Work out the finished part from the listing and answer in its coordinate system (mm). Give positions to 0.01 mm unless a question says otherwise; leave off trailing zeros. Loops run counter-clockwise (first coordinate to the right, second up) from the corner with the lowest first, then second, coordinate; pieces in that order, holes last. Notation, with made-up numbers: M 64.25,-34 L 99.25,-34 A12 cw 99.25,-29 Z; hole C 23,12 d1. An arc over 180 degrees is marked long. Use a Markdown table: item, result.
```python
from build123d import *

# Parameters (mm, degrees)
SKETCH1_R               = 19.05
BOSS_EXTRUDE1_DEPTH     = 1524
SHELL1_T                = -2.54
CUT_EXTRUDE1_DEPTH      = 127
CUT_EXTRUDE1_DEPTH_BACK = 127
SKETCH2_OUTSIDE_W       = 1830.99
SKETCH2_OUTSIDE_H       = 345.09


with BuildPart() as part:
    # Sketch1 → Boss-Extrude1 (new body)
    with BuildSketch(Plane.XY):
        Circle(SKETCH1_R)
    extrude(amount=BOSS_EXTRUDE1_DEPTH)

    # Shell1
    shell1_openings = [part.faces().sort_by_distance(p)[0] for p in [
        (0, 0, 0),
    ]]
    offset(amount=SHELL1_T, openings=shell1_openings, kind=Kind.INTERSECTION)

    # Sketch2 outside → Cut-Extrude1 (cut, two sides: drawn at the far end of the back side and taken through both)
    with BuildSketch(Plane(origin=(0, 0, 0), x_dir=(0, 0, -1), z_dir=(1, 0, 0)).offset(-CUT_EXTRUDE1_DEPTH_BACK)):
        with Locations((-762, 0)):
            Rectangle(SKETCH2_OUTSIDE_W, SKETCH2_OUTSIDE_H)
        Polygon((-1524, -76.2), (-1368.114799795, 76.2), (0, 76.2), (0, -76.2), align=None, mode=Mode.SUBTRACT)
    extrude(amount=CUT_EXTRUDE1_DEPTH + CUT_EXTRUDE1_DEPTH_BACK, mode=Mode.SUBTRACT)


solid = part.part
```
(1) Given P1, Ø3, axis at y = 14, z = 395, coming from the +X side; P2, Ø1, axis at y = 3.5, z = 891, coming from the +X side; P3, Ø1, axis at y = -9.5, z = 268, coming from the -X side, each flat-ended and moving along its own axis, determine where each tip first touches the part or whether it passes through.
Entries:
| item | result |
|---|---|
| P1 | stops at x = 14.38 |
| P2 | stops at x = 18.81 |
| P3 | stops at x = -16.79 |
(2) The mould has two halves that part along X. Classify faces 1 (the flat face through (-17.02, -0.09, 1446.15)), 2 (the cylindrical face through (15.748, 4.959, 721.399)), 3 (the cylindrical face through (-15.12, -11.59, 722.71)): released by +X, released by -X, zero draft, split by the parting line, or undercut.
Entries:
| item | result |
|---|---|
| face 1 | zero draft |
| face 2 | undercut |
| face 3 | split by the parting line |
(3) A cutting plane is placed at C-C (z = 1193.5). Write down the section's boundary in (x, y).
Entries:
| item | result |
|---|---|
| outline | C 0,0 d38.1; hole C 0,0 d33.02 |
(4) A cutting plane is placed at A-A (x = 0). Write down the section's boundary in (y, z).
Entries:
| item | result |
|---|---|
| outline | M -19.05,0 L -16.51,0 L -16.51,1462.94 L -19.05,1465.54 Z; M 16.51,0 L 19.05,0 L 19.05,1426.57 L 16.51,1429.17 Z |
(5) A cutting plane is placed at B-B (y = 0). Write down the section's boundary in (x, z).
Entries:
| item | result |
|---|---|
| outline | M -19.05,0 L -16.51,0 L -16.51,1446.06 L -19.05,1446.06 Z; M 16.51,0 L 19.05,0 L 19.05,1446.06 L 16.51,1446.06 Z |
(6) Consider probe 1 along Y at (x, z) = (0, 970); probe 2 along X at (y, z) = (-2.5, 441.5). Determine where each line is inside the solid, lowest interval first. Write a range as [from, to].
Entries:
| item | result |
|---|---|
| probe 1 | y = [-19.05, -16.51], [16.51, 19.05] |
| probe 2 | x = [-18.89, -16.32], [16.32, 18.89] |
